The model under review builds one solid part; all positions refer to its coordinate system, in mm. A direction names the side the tool comes from. Round coordinates to 2 decimals unless told otherwise and drop trailing zeros. Order: outer loops, then holes, each group sorted by start corner. A loop starts at its lowest first (then second) coordinate and runs counter-clockwise, first axis right, second up. Notation, with made-up numbers: (73.5, -15) -> (111.5, -15) arc R29 cw to (111.5, 16) -> close; hole circle Ø5 at (76.25, -13.75). An arc over 180 degrees is marked (long way). Return JSON: item names as keys, results as strings. Group by question number.
Autodesk Inventor part; units mm, degrees
ref_plane "YZ Plane" through (0, 0, 0) normal (1, 0, 0) x (0, 1, 0)
ref_plane "XZ Plane" through (0, 0, 0) normal (0, 1, 0) x (-1, 0, 0)
ref_plane "XY Plane" through (0, 0, 0) normal (0, 0, 1) x (1, 0, 0)
sketch "Sketch1" plane through (0, 0, 0) normal (0, 1, 0) x (-1, 0, 0)
  line L0 (-27.94, 42.8625) -> (-31.75, 42.8625)
  line L1 (-31.75, 42.8625) -> (-31.75, 23.8125)
  line L2 (-31.75, 23.8125) -> (-27.94, 23.8125)
  line L3 (-27.94, 23.8125) -> (-27.94, 42.8625)
  line L4 (-27.94, 38.1) -> (-24.765, 38.1)
  line L5 (-24.765, 38.1) -> (-24.765, 28.575)
  line L6 (-24.765, 28.575) -> (-27.94, 28.575)
  line L7 (-27.94, 28.575) -> (-27.94, 38.1)
  line L8 (-31.75, 38.1) -> (-28.575, 38.1)
  line L9 (-28.575, 28.575) -> (-31.75, 28.575)
  line L10 (-31.75, 28.575) -> (-31.75, 38.1)
  line L11 (-28.575, 28.575) -> (-31.75, 28.575)
  line L12 (-31.75, 28.575) -> (-31.75, 23.8125)
  line L13 (-31.75, 23.8125) -> (-28.575, 23.8125)
  line L14 (-28.575, 23.8125) -> (-28.575, 28.575)
  line L15 (-28.575, 38.1) -> (-31.75, 38.1)
  line L16 (-31.75, 38.1) -> (-31.75, 42.8625)
  line L17 (-31.75, 42.8625) -> (-28.575, 42.8625)
  line L18 (-28.575, 42.8625) -> (-28.575, 38.1)
  point P0 (0, 0)
  dimension "d0" = 4.7625
  dimension "d1" = 4.7625
  dimension "d2" = 19.05
  dimension "d3" = 3.175
  dimension "d4" = 3.81
extrude "Extrusion2" add sketch "Sketch1" along normal blind 3.175 contours L3 L2 L14 L9 L1 L8 L18 L0 | L4 L5 L6 L3
Item 1: Wall thickness on line 1 along X through (y, z) = (2.9, 41.25) (3 decimals); line 2 along Z through (x, y) = (31, 0.95) (3 decimals): over which ranges is each line inside the solid? List them lowest first.
Item 2: Insertion check: pin 1 Ø1 at (x, y) = (25.5, 2.5) entering from +Z; pin 2 Ø1 at (y, z) = (2, 27) entering from -X; pin 3 Ø1.6 at (x, y) = (30.5, 1) entering from -Z (3 decimals). Each pin has a flat end and moves straight along its axis. Give the tip position at first contact, or say it passes through.
Item 3: For faces 1 (the face through (28.575, 2, 26)), 2 (the face through (28, 0, 33)), 3 (the face through (27.94, 2, 40)), 4 (the face through (28.575, 2, 41)), 5 (the face through (26, 2, 28.575)), list the 3-axis set-ups (+Z, -Z, +X, -X, +Y, -Y) from which the entire face can be reached by the end or side of a thin tool; tool diameter is ignored.
Item 4: Consider section B-B on x = 28.75. State the section outline as (y, z) points (3 decimals).
Item 5: Consider section C-C on z = 39.75. State the section outline as (x, y) points (3 decimals), plus the area to 3 significant figures.
Values:
{
 "1": {"line 1": "27.94 to 28.575", "line 2": "28.575 to 38.1"},
 "2": {"pin 1": "z = 38.1", "pin 2": "x = 27.94", "pin 3": "z = 28.575"},
 "3": {"face 1": "-Z, +X, +Y, -Y", "face 2": "+Z, -Z, +X, -X, -Y", "face 3": "+Z, -X, +Y, -Y", "face 4": "+Z, +X, +Y, -Y", "face 5": "-Z, -X, +Y, -Y"},
 "4": {"outline": "(0, 28.575) -> (3.175, 28.575) -> (3.175, 38.1) -> (0, 38.1) -> close"},
 "5": {"outline": "(27.94, 0) -> (28.575, 0) -> (28.575, 3.175) -> (27.94, 3.175) -> close", "area": "2.02 mm^2"}
}
